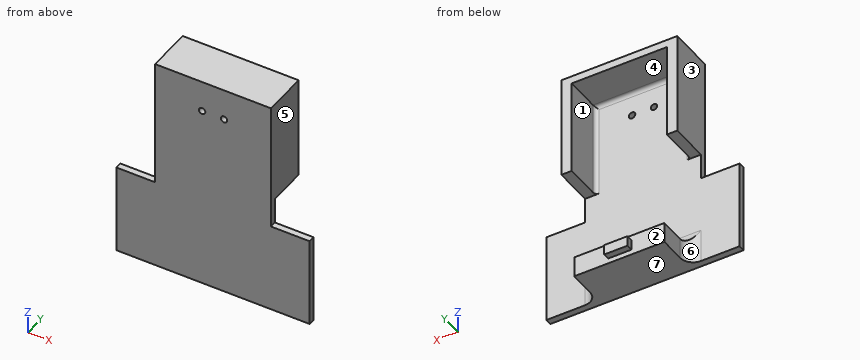
from build123d import *

# Parameters (mm, degrees)
SKETCH1_R           = 2.5
BOSS_EXTRUDE1_DEPTH = 5
SKETCH2_W           = 70
SKETCH2_H           = 16
BOSS_EXTRUDE2_DEPTH = 30
FILLET1_R           = 10
FILLET2_R           = 3
SKETCH9_W           = 18
SKETCH9_H           = 8
BOSS_EXTRUDE9_DEPTH = 5


with BuildPart() as part:
    # Sketch1 → Boss-Extrude1 (new body)
    with BuildSketch(Plane(origin=(0, 0, 0), x_dir=(1, 0, 0), z_dir=(0, 1, 0))):
        Polygon((-45, -85), (45, -85), (45, 15), (75, 15), (75, 85), (-75, 85), (-75, 15), (-45, 15), align=None)
        with Locations(Location((-8.5, -60.45079013, 0), (0, 0, 270))):
            Circle(SKETCH1_R, mode=Mode.SUBTRACT)
        with Locations(Location((8.5, -60.45079013, 0), (0, 0, 270))):
            Circle(SKETCH1_R, mode=Mode.SUBTRACT)
    extrude(amount=BOSS_EXTRUDE1_DEPTH)

    # Sketch2 → Boss-Extrude2 (add)
    with BuildSketch(Plane(origin=(0, 5, 0), x_dir=(1, 0, 0), z_dir=(0, 1, 0))):
        Polygon((-45, -85), (-25, -85), (25, -85), (45, -85), (45, -76.441120724), (45, -5), (37, -5), (37, -79), (-37, -79), (-37, -5), (-45, -5), (-45, -76.441120724), align=None)
        with Locations((0, 77)):
            Rectangle(SKETCH2_W, SKETCH2_H)
    extrude(amount=BOSS_EXTRUDE2_DEPTH)

    # Fillet1
    fillet1_edges = [part.edges().sort_by_distance(p)[0] for p in [
        (0, 5, -69),
        (35, 5, -77),
        (-35, 5, -77),
    ]]
    fillet(fillet1_edges, radius=FILLET1_R)

    # Fillet2
    fillet2_edges = [part.edges().sort_by_distance(p)[0] for p in [
        (37, 5, 42),
        (0, 5, 79),
        (-37, 5, 42),
    ]]
    fillet(fillet2_edges, radius=FILLET2_R)

    # Sketch9 → Boss-Extrude9 (add)
    with BuildSketch(Plane(origin=(0, 35, 0), x_dir=(1, 0, 0), z_dir=(0, 1, 0))):
        with Locations((-0.264957407, 76.945272118)):
            Rectangle(SKETCH9_W, SKETCH9_H)
    extrude(amount=BOSS_EXTRUDE9_DEPTH)


solid = part.part
Input: part model. Units: mm. Frame: model coordinates. Face numbers are marked on the shaded views. A direction names the side the tool comes from. Give positions to 0.01 mm unless a question says otherwise; leave off trailing zeros. Write each loop counter-clockwise with the first axis right and the second up, starting at its lowest first coordinate (ties: lowest second). Pieces come first, ordered by that corner, then holes. Notation, with made-up numbers: M 28,67 L 84,67 A33 cw 84,97 Z; hole C 47.5,55.5 d5. An arc over 180 degrees is marked long. Write item = value, one per line. Start each with the question number.
1) Cut plane A-A on y = 30.5. Return the cut outline in (x, z), then the cut area to 3 significant figures.
2) Cut plane D-D on z = -6.5. Return the cut outline in (x, y).
3) Reachability of the marked faces 4, 5, 6 and 7 from +Z, -Z, +X, -X, +Y, -Y: full face, straight path, thin tool, end or side. Return the list, or none.
4) Cut plane B-B on x = 17.5. Return the cut outline in (y, z), then the cut area to 3 significant figures.
5) Cut plane C-C on z = 68. Return the cut outline in (x, y), then the cut area to 3 significant figures.
6) Material intervals for line 1 along X through (y, z) = (20, 20.5); line 2 along Z through (x, y) = (26, 23); line 3 along Y through (x, z) = (19, 58.5), sorted ascending. Write a range as [from, to].
7) Draft query along X for the marked faces 1, 2 and 3. Return one class per face: +X half, -X half, draft (parallel to the pull), parting line (faces both ways), or undercut.
8) First-contact query: pin 1 Ø3.5 at (x, y) = (-39.5, 21) entering from -Z; pin 2 Ø1.5 at (x, z) = (-56, -24.5) entering from +Y; pin 3 Ø2.5 at (x, y) = (-62.5, 3.5) entering from +Z. Flat tips, straight axial feed; report the tip coordinate or a pass-through.
Solved:
q1.outline = M -45,5 L -37,5 L -37,79 L 37,79 L 37,5 L 45,5 L 45,85 L -45,85 Z; M -35,-85 L 35,-85 L 35,-69 L -35,-69 Z
q1.area = 2,840 mm2
q2.outline = M -45,0 L 45,0 L 45,5 L -45,5 Z
q3.face_4 = +Y
q3.face_5 = +Z, +X, +Y, -Y
q3.face_6 = -Z, -X, +Y
q3.face_7 = -Z, +X, -X, +Y, -Y
q4.outline = M 0,-85 L 35,-85 L 35,-69 L 15,-69 A10 cw 5,-59 L 5,76 A3 cw 8,79 L 35,79 L 35,85 L 0,85 Z
q4.area = 1,530 mm2
q5.outline = M -45,0 L 45,0 L 45,35 L 37,35 L 37,8 A3 cw 34,5 L -34,5 A3 cw -37,8 L -37,35 L -45,35 Z
q5.area = 934 mm2
q6.line_1 = [-45, -37], [37, 45]
q6.line_2 = [-85, -69], [79, 85]
q6.line_3 = [0, 5]
q7.face_1 = undercut
q7.face_2 = draft
q7.face_3 = -X half
q8.pin_1 = 5
q8.pin_2 = 5
q8.pin_3 = -15
